```python
from build123d import *

# Parameters (mm, degrees)
SKETCH1_W               = 80
SKETCH1_H               = 281.62
BOSS_EXTRUDE1_DEPTH     = 2
SKETCH2_R               = 1.85
CUT_EXTRUDE1_DEPTH      = 2
SKETCH3_R               = 1.25
CUT_EXTRUDE2_DEPTH      = 2
LPATTERN1_COUNT         = 3
LPATTERN1_PITCH         = 66.76
MIRROR1_COPY_1_SKETCH_R = 1.25
MIRROR1_COPY_1_DEPTH    = 2
MIRROR1_COPY_2_SKETCH_R = 1.25
MIRROR1_COPY_2_DEPTH    = 2
SKETCH4_R               = 2.5
CUT_EXTRUDE3_DEPTH      = 10


with BuildPart() as part:
    # Sketch1 → Boss-Extrude1 (new body)
    with BuildSketch(Plane(origin=(0, 0, 0), x_dir=(1, 0, 0), z_dir=(0, 1, 0))):
        Rectangle(SKETCH1_W, SKETCH1_H)
    extrude(amount=BOSS_EXTRUDE1_DEPTH)

    # Sketch2 → Cut-Extrude1 (cut)
    with BuildSketch(Plane(origin=(0, 2, 0), x_dir=(1, 0, 0), z_dir=(0, 1, 0))):
        with Locations(Location((0, 135.87, 0), (0, 0, 270))):
            Circle(SKETCH2_R)
    extrude(amount=-CUT_EXTRUDE1_DEPTH, mode=Mode.SUBTRACT)

    # Sketch3 → Cut-Extrude2 (cut)
    with BuildSketch(Plane(origin=(0, 2, 0), x_dir=(1, 0, 0), z_dir=(0, 1, 0))):
        with Locations(Location((-36, 68.81, 0), (0, 0, 270))):
            Circle(SKETCH3_R)
    cut_extrude2 = extrude(amount=-CUT_EXTRUDE2_DEPTH, mode=Mode.SUBTRACT)

    # LPattern1: Cut-Extrude2 ×3
    with Locations(*[(0, 0, i * LPATTERN1_PITCH) for i in range(1, LPATTERN1_COUNT)]):
        add(cut_extrude2, mode=Mode.SUBTRACT)

    # Mirror1: Cut-Extrude2 across plane
    add(cut_extrude2.mirror(Plane(origin=(0, 0, 0), x_dir=(0, 0, 1), z_dir=(1, 0, 0))), mode=Mode.SUBTRACT)

    # Mirror1 copy 1 sketch → Mirror1 copy 1 (cut)
    with BuildSketch(Plane(origin=(0, 2, 66.76), x_dir=(-1, 0, 0), z_dir=(0, 1, 0))):
        with Locations((-36, -68.81)):
            Circle(MIRROR1_COPY_1_SKETCH_R)
    extrude(amount=-MIRROR1_COPY_1_DEPTH, mode=Mode.SUBTRACT)

    # Mirror1 copy 2 sketch → Mirror1 copy 2 (cut)
    with BuildSketch(Plane(origin=(0, 2, 133.52), x_dir=(-1, 0, 0), z_dir=(0, 1, 0))):
        with Locations((-36, -68.81)):
            Circle(MIRROR1_COPY_2_SKETCH_R)
    extrude(amount=-MIRROR1_COPY_2_DEPTH, mode=Mode.SUBTRACT)

    # Sketch4 → Cut-Extrude3 (cut)
    with BuildSketch(Plane(origin=(0, 2, 0), x_dir=(1, 0, 0), z_dir=(0, 1, 0))):
        with Locations(Location((0, 105.81, 0), (0, 0, 270))):
            Circle(SKETCH4_R)
    cut_extrude3 = extrude(amount=-CUT_EXTRUDE3_DEPTH, mode=Mode.SUBTRACT)

    # Mirror2: Cut-Extrude3 across plane
    add(cut_extrude3.mirror(Plane.XY), mode=Mode.SUBTRACT)


solid = part.part
```
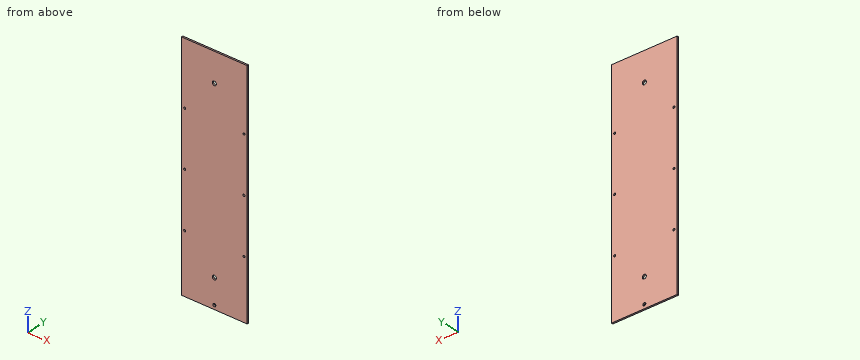
Read the model definition and answer for the solid it produces. Units are mm, in the model's axes. Give positions to 0.01 mm unless a question says otherwise; leave off trailing zeros. Order: outer loops, then holes, each group sorted by start corner. A loop starts at its lowest first (then second) coordinate and runs counter-clockwise, first axis right, second up.
(1) Given pin 1 (1.5 mm diameter, centred on x = 36, z = -2.05, fed in from -Y); pin 2 (5 mm diameter, centred on x = -29, z = 102, fed in from -Y), each flat-ended and moving along its own axis, determine where each tip first touches the part or whether it passes through.
(2) Straight lines are drawn through the part: L1, parallel to X at y = 1.55, z = -68.81; L2, parallel to Z at x = 36, y = 0.6; L3, parallel to X at y = 1, z = 105.81. For each, find the intervals that lie inside material, in ascending order.
(3) Find section A-A (z = 105.81). Give the vertices of the cut face in (x, y), plus the area to 3 significant figures.
Result sheet:
1. pin 1: passes through
1. pin 2: stops at y = 0
2. L1: x = -40 to -37.25, -34.75 to 34.75, 37.25 to 40
2. L2: z = -140.81 to -70.06, -67.56 to -3.3, -0.8 to 63.46, 65.96 to 140.81
2. L3: x = -40 to -2.5, 2.5 to 40
3. outline: (-40, 0) - (-2.5, 0) - (-2.5, 2) - (-40, 2) - close; (2.5, 0) - (40, 0) - (40, 2) - (2.5, 2) - close
3. area: 150 mm2
